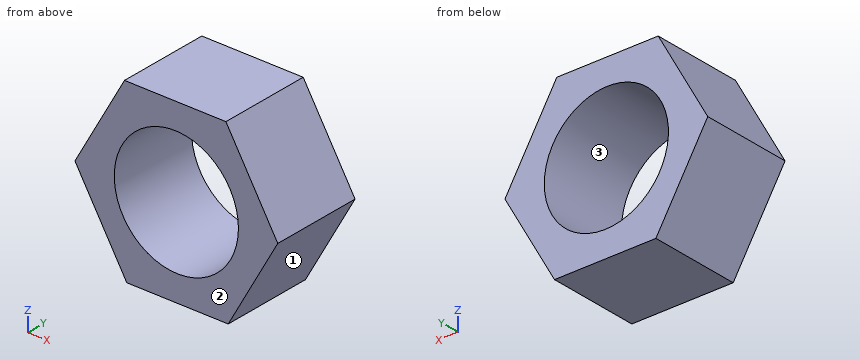
```python
from build123d import *

# Parameters (mm, degrees)
F0_R     = 17.482868
F1_DEPTH = 25.4
F2_DEPTH = 25.4


with BuildPart() as f1:
    # F0 (on Front) → F1 (new body)
    with BuildSketch(Plane.XZ):
        Polygon((-14.606514, 24.550197), (-28.564351, -0.374514), (-13.957837, -24.924711), (14.606514, -24.550197), (28.564351, 0.374514), (13.957837, 24.924711), align=None)
        Circle(F0_R, mode=Mode.SUBTRACT)
    extrude(amount=F1_DEPTH)

    # F0 (on Front) → F2 (join)
    with BuildSketch(Plane.XZ):
        Polygon((-14.606514, 24.550197), (-28.564351, -0.374514), (-13.957837, -24.924711), (14.606514, -24.550197), (28.564351, 0.374514), (13.957837, 24.924711), align=None)
        Circle(F0_R, mode=Mode.SUBTRACT)
    extrude(amount=F2_DEPTH)


solid = f1.part
```
Input: part model. Units: mm. Frame: model coordinates. Face numbers are marked on the shaded views. Give positions to 0.01 mm unless a question says otherwise; leave off trailing zeros. Loops run counter-clockwise (first coordinate to the right, second up) from the corner with the lowest first, then second, coordinate; pieces in that order, holes last.
1) Mould query, pull axis X, two halves, no side actions, for the marked faces 1, 2 and 3. Classes: released by +X, released by -X, zero draft, split by the parting line, or undercut.
A:
face 1: released by +X
face 2: zero draft
face 3: undercut
2) Line query: L1, parallel to Z at x = 0, y = -6.25; L2, parallel to Z at x = 8.5, y = -18.25; L3, parallel to X at y = -16, z = 4.5. Output: solid intervals per line, ascending.
A:
L1: z = -24.74 to -17.48, 17.48 to 24.74
L2: z = -24.63 to -15.28, 15.28 to 24.85
L3: x = -25.83 to -16.89, 16.89 to 26.11
3) Section query B-B on x = 11. Return the cut outline in (y, z), and give its area (3 significant figures).
A:
outline: (-25.4, -24.6) - (0, -24.6) - (0, -13.59) - (-25.4, -13.59) - close; (-25.4, 13.59) - (0, 13.59) - (0, 24.89) - (-25.4, 24.89) - close
area: 567 mm2
4) Section query C-C on z = -12. Return the cut outline in (x, y), and give its area (3 significant figures).
A:
outline: (-21.65, -25.4) - (-12.71, -25.4) - (-12.71, 0) - (-21.65, 0) - close; (12.71, -25.4) - (21.63, -25.4) - (21.63, 0) - (12.71, 0) - close
area: 453 mm2
5) Section query D-D on x = 20.5. Return the cut outline in (y, z), and give its area (3 significant figures).
A:
outline: (-25.4, -14.03) - (0, -14.03) - (0, 13.93) - (-25.4, 13.93) - close
area: 710 mm2
6) Section query A-A on y = -16.75. Return the cut outline in (x, z), and give its area (3 significant figures).
A:
outline: (-28.56, -0.37) - (-13.96, -24.92) - (14.61, -24.55) - (28.56, 0.37) - (13.96, 24.92) - (-14.61, 24.55) - close; hole circle Ø34.97 at (0, 0)
area: 1,160 mm2
7) Contact query for flat-ended pins moving along their axis: pin 1 (6 mm diameter, centred on y = -6, z = -19, fed in from +X); pin 2 (8 mm diameter, centred on x = -13.5, z = -4.5, fed in from +Y); pin 3 (6 mm diameter, centred on y = -8.5, z = 8.5, fed in from +X); pin 4 (8 mm diameter, centred on y = -15.5, z = 16, fed in from +X). Output: stop coordinate, or through.
A:
pin 1: stops at x = 19.39
pin 2: stops at y = 0
pin 3: stops at x = 25.51
pin 4: stops at x = 21.65
